Part model, mm, in its own coordinate system. A direction names the side the tool comes from. Round coordinates to 2 decimals unless told otherwise and drop trailing zeros. Loops run counter-clockwise (first coordinate to the right, second up) from the corner with the lowest first, then second, coordinate; pieces in that order, holes last. Notation, with made-up numbers: (52.25, -18.5) - (75.25, -18.5) arc R9 cw to (75.25, -8.5) - close; hole circle Ø9 at (1.5, 0). An arc over 180 degrees is marked (long way). Put each result on its own line as item: value.
from build123d import *

# Parameters (mm, degrees)
ESQUISSE2_W             = 173.5
ESQUISSE2_H             = 80
BOSS_EXTRU_2_DEPTH      = 3
ENL_V_MAT_EXTRU_1_REACH = 193.079
ESQUISSE3_W             = 3
ESQUISSE3_H             = 20
ESQUISSE4_W             = 20
ESQUISSE4_H             = 3
BOSS_EXTRU_3_DEPTH      = 3
ESQUISSE5_W             = 4
ESQUISSE5_H             = 20
ENL_V_MAT_EXTRU_2_DEPTH = 10
ESQUISSE6_W             = 20
ESQUISSE6_H             = 24
ENL_V_MAT_EXTRU_3_DEPTH = 10


with BuildPart() as part:
    # Esquisse2 → Boss.-Extru.2 (new body)
    with BuildSketch(Plane.XY):
        with Locations((-86.75, -40)):
            Rectangle(ESQUISSE2_W, ESQUISSE2_H)
    extrude(amount=BOSS_EXTRU_2_DEPTH)

    # Esquisse3 → Enlèv. mat.-Extru.1 (cut, up to next)
    with BuildSketch(Plane.XY.offset(3), mode=Mode.PRIVATE) as enl_v_mat_extru_1_sk1:
        with Locations((-51.5, -60)):
            Rectangle(ESQUISSE3_W, ESQUISSE3_H)
    enl_v_mat_extru_1_tool1 = extrude(enl_v_mat_extru_1_sk1.sketch, amount=-ENL_V_MAT_EXTRU_1_REACH, mode=Mode.PRIVATE) & part.part
    # Esquisse3 → Enlèv. mat.-Extru.1 (cut, up to next)
    with BuildSketch(Plane.XY.offset(3), mode=Mode.PRIVATE) as enl_v_mat_extru_1_sk2:
        with Locations((-51.5, -20)):
            Rectangle(ESQUISSE3_W, ESQUISSE3_H)
    enl_v_mat_extru_1_tool2 = extrude(enl_v_mat_extru_1_sk2.sketch, amount=-ENL_V_MAT_EXTRU_1_REACH, mode=Mode.PRIVATE) & part.part
    add(enl_v_mat_extru_1_tool1.solids().sort_by_distance((-51.5, -60, 3))[0], mode=Mode.SUBTRACT)
    add(enl_v_mat_extru_1_tool2.solids().sort_by_distance((-51.5, -20, 3))[0], mode=Mode.SUBTRACT)

    # Esquisse4 → Boss.-Extru.3 (add)
    with BuildSketch(Plane(origin=(0, 0, 0), x_dir=(1, 0, 0), z_dir=(0, 1, 0))):
        with Locations((-96.75, -1.5)):
            Rectangle(ESQUISSE4_W, ESQUISSE4_H)
    extrude(amount=BOSS_EXTRU_3_DEPTH)

    # Esquisse5 → Enlèv. mat.-Extru.2 (cut)
    with BuildSketch(Plane(origin=(0, 0, 0), x_dir=(-1, 0, 0), z_dir=(0, 0, -1))):
        with Locations((7, -40)):
            Rectangle(ESQUISSE5_W, ESQUISSE5_H)
    extrude(amount=-ENL_V_MAT_EXTRU_2_DEPTH, mode=Mode.SUBTRACT)

    # Esquisse6 → Enlèv. mat.-Extru.3 (cut)
    with BuildSketch(Plane.XY.offset(3)):
        with Locations((-163.5, -38)):
            Rectangle(ESQUISSE6_W, ESQUISSE6_H)
    extrude(amount=-ENL_V_MAT_EXTRU_3_DEPTH, mode=Mode.SUBTRACT)


solid = part.part
1. Band-saw the part on A-A (y = -64). List the corners of the cut face in (x, z).
A:
outline: (-173.5, 0) - (-53, 0) - (-53, 3) - (-173.5, 3) - close; (-50, 0) - (0, 0) - (0, 3) - (-50, 3) - close
2. Tool access for faces 1 (the flat face through (-173.5, -13, 1)), 2 (the flat face through (-7, -30, 1)), 3 (the flat face through (-164, -26, 2)), 4 (the flat face through (-141, 0, 1)), 5 (the flat face through (-97, 3, 1)): list every direction of +Z, -Z, +X, -X, +Y, -Y with a clear straight run to the whole face (end or side of a thin tool).
A:
face 1: +Z, -Z, -X, +Y, -Y
face 2: +Z, -Z
face 3: +Z, -Z, -X
face 4: +Z, -Z, -X, +Y
face 5: +Z, -Z, +X, -X, +Y
3. Band-saw the part on B-B (z = 2.4). List the corners of the cut face in (x, y).
A:
outline: (-173.5, -80) - (0, -80) - (0, 0) - (-86.75, 0) - (-86.75, 3) - (-106.75, 3) - (-106.75, 0) - (-173.5, 0) - (-173.5, -26) - (-153.5, -26) - (-153.5, -50) - (-173.5, -50) - close; hole (-53, -70) - (-50, -70) - (-50, -50) - (-53, -50) - close; hole (-53, -30) - (-50, -30) - (-50, -10) - (-53, -10) - close; hole (-9, -50) - (-5, -50) - (-5, -30) - (-9, -30) - close
4. Band-saw the part on C-C (x = -31). List the corners of the cut face in (y, z).
A:
outline: (-80, 0) - (0, 0) - (0, 3) - (-80, 3) - close
5. Two-plate mould, pull along Y, no slides. Class faces 6 (the flat face through (-106.75, 1, 2)), 7 (the flat face through (-164, -50, 2)), 8 (the flat face through (-44, 0, 1)): pulls with the +Y half, pulls with the -Y half, needs draft (parallel to the pull), parting line crosses it, or undercut.
A:
face 6: needs draft
face 7: undercut
face 8: pulls with the +Y half
6. Probe line 1 along X through (y, z) = (-16, 0.3); line 2 along Y through (x, z) = (-162.5, 0.45); line 3 along Y through (x, z) = (-85, 0.65). List the from-to ranges inside material, lowest first. Write a range as [from, to].
A:
line 1: x = [-173.5, -53], [-50, 0]
line 2: y = [-80, -50], [-26, 0]
line 3: y = [-80, 0]
7. Pin check, flat tips, straight feed: P1, Ø1.5, axis at x = -51.5, z = 1.5, coming from the +Y side; P2, Ø0.9, axis at y = -32.5, z = 1, coming from the -X side; P3, Ø0.9, axis at y = 2, z = 2, coming from the -X side. Stop position of each tip, or through.
A:
P1: stops at y = 0
P2: stops at x = -153.5
P3: stops at x = -106.75
